Geometry check sheet. Reference: the model listing, model coordinates, mm. Face numbers are marked on the shaded views. A direction names the side the tool comes from. Coordinates: 2 decimals unless noted, no trailing zeros. Loops run counter-clockwise (first coordinate to the right, second up) from the corner with the lowest first, then second, coordinate; pieces in that order, holes last. Notation, with made-up numbers: (42.5, -15) -> (48.5, -15) arc R25 ccw to (48.5, -3) -> close; hole circle Ø1 at (-23.75, -13.75). An arc over 180 degrees is marked (long way). Answer as a JSON object with one key per item and string values.
from build123d import *

# Parameters (mm, degrees)
F0_W     = 440
F0_H     = 440
F1_DEPTH = 50.8
F0_W_2   = 50.8
F0_H_2   = 203.2
F0_W_3   = 203.2
F0_H_3   = 50.8
F2_DEPTH = 349.2
F3_DEPTH = 149.2
F4_W     = 440
F4_H     = 440
F4_W_2   = 50.8
F4_H_2   = 50.8
F5_DEPTH = 200


# Not quite as in the source:
# - a feature names something its author has since deleted; it is built from what else it names


with BuildPart() as f1:
    # F0 (on Top) → F1 (new body)
    with BuildSketch(Plane.XY):
        Polygon((91.7435496044, 289.8852448295), (-163.4564503956, 289.8852448295), (-163.4564503956, 239.0852448295), (-163.4564503956, 35.8852448295), (-214.2564503956, 35.8852448295), (-214.2564503956, -219.3147551705), (-163.4564503956, -219.3147551705), (39.7435496044, -219.3147551705), (39.7435496044, -270.1147551705), (294.9435496044, -270.1147551705), (294.9435496044, -219.3147551705), (294.9435496044, -16.1147551705), (345.7435496044, -16.1147551705), (345.7435496044, 239.0852448295), (294.9435496044, 239.0852448295), (91.7435496044, 239.0852448295), align=None)
        with Locations((65.7435496044, 9.8852448295)):
            Rectangle(F0_W, F0_H, mode=Mode.SUBTRACT)
        with Locations((65.7435496044, 9.8852448295)):
            Rectangle(F0_W, F0_H)
        Polygon((-65.0564503956, 140.6852448295), (-14.2564503956, 140.6852448295), (87.3435496044, 140.6852448295), (196.5435496044, 140.6852448295), (196.5435496044, 89.8852448295), (196.5435496044, -11.7147551705), (196.5435496044, -120.9147551705), (145.7435496044, -120.9147551705), (44.1435496044, -120.9147551705), (-65.0564503956, -120.9147551705), (-65.0564503956, -70.1147551705), (-65.0564503956, 31.4852448295), align=None, mode=Mode.SUBTRACT)
        Polygon((87.3435496044, 89.8852448295), (-14.2564503956, 89.8852448295), (-14.2564503956, 140.6852448295), (-65.0564503956, 140.6852448295), (-65.0564503956, 31.4852448295), (-14.2564503956, 31.4852448295), (-14.2564503956, -70.1147551705), (-65.0564503956, -70.1147551705), (-65.0564503956, -120.9147551705), (44.1435496044, -120.9147551705), (44.1435496044, -70.1147551705), (145.7435496044, -70.1147551705), (145.7435496044, -120.9147551705), (196.5435496044, -120.9147551705), (196.5435496044, -11.7147551705), (145.7435496044, -11.7147551705), (145.7435496044, 89.8852448295), (196.5435496044, 89.8852448295), (196.5435496044, 140.6852448295), (87.3435496044, 140.6852448295), align=None)
    extrude(amount=-F1_DEPTH)

    # F0 (on Top) → F2 (join)
    with BuildSketch(Plane.XY):
        Polygon((91.7435496044, 289.8852448295), (-163.4564503956, 289.8852448295), (-163.4564503956, 239.0852448295), (-163.4564503956, 35.8852448295), (-214.2564503956, 35.8852448295), (-214.2564503956, -219.3147551705), (-163.4564503956, -219.3147551705), (39.7435496044, -219.3147551705), (39.7435496044, -270.1147551705), (294.9435496044, -270.1147551705), (294.9435496044, -219.3147551705), (294.9435496044, -16.1147551705), (345.7435496044, -16.1147551705), (345.7435496044, 239.0852448295), (294.9435496044, 239.0852448295), (91.7435496044, 239.0852448295), align=None)
        with Locations((65.7435496044, 9.8852448295)):
            Rectangle(F0_W, F0_H, mode=Mode.SUBTRACT)
        with Locations((320.3435496044, -117.7147551705)):
            Rectangle(F0_W_2, F0_H_2)
        with Locations((193.3435496044, 264.4852448295)):
            Rectangle(F0_W_3, F0_H_3)
        with Locations((-188.8564503956, 137.4852448295)):
            Rectangle(F0_W_2, F0_H_2)
        with Locations((-61.8564503956, -244.7147551705)):
            Rectangle(F0_W_3, F0_H_3)
    extrude(amount=F2_DEPTH)

    # F0 (on Top) → F3 (join)
    with BuildSketch(Plane.XY):
        with Locations((65.7435496044, 9.8852448295)):
            Rectangle(F0_W, F0_H)
        Polygon((-65.0564503956, 140.6852448295), (-14.2564503956, 140.6852448295), (87.3435496044, 140.6852448295), (196.5435496044, 140.6852448295), (196.5435496044, 89.8852448295), (196.5435496044, -11.7147551705), (196.5435496044, -120.9147551705), (145.7435496044, -120.9147551705), (44.1435496044, -120.9147551705), (-65.0564503956, -120.9147551705), (-65.0564503956, -70.1147551705), (-65.0564503956, 31.4852448295), align=None, mode=Mode.SUBTRACT)
        Polygon((87.3435496044, 89.8852448295), (-14.2564503956, 89.8852448295), (-14.2564503956, 140.6852448295), (-65.0564503956, 140.6852448295), (-65.0564503956, 31.4852448295), (-14.2564503956, 31.4852448295), (-14.2564503956, -70.1147551705), (-65.0564503956, -70.1147551705), (-65.0564503956, -120.9147551705), (44.1435496044, -120.9147551705), (44.1435496044, -70.1147551705), (145.7435496044, -70.1147551705), (145.7435496044, -120.9147551705), (196.5435496044, -120.9147551705), (196.5435496044, -11.7147551705), (145.7435496044, -11.7147551705), (145.7435496044, 89.8852448295), (196.5435496044, 89.8852448295), (196.5435496044, 140.6852448295), (87.3435496044, 140.6852448295), align=None)
    extrude(amount=F3_DEPTH)

    # F4 (on face) → F5 (join)
    with BuildSketch(Plane.XY.offset(349.2)):
        Polygon((-163.4564503956, -219.3147551705), (-163.4564503956, -270.1147551705), (294.9435496044, -270.1147551705), (294.9435496044, -219.3147551705), (345.7435496044, -219.3147551705), (345.7435496044, 239.0852448295), (294.9435496044, 239.0852448295), (294.9435496044, 289.8852448295), (-163.4564503956, 289.8852448295), (-163.4564503956, 239.0852448295), (-214.2564503956, 239.0852448295), (-214.2564503956, -219.3147551705), align=None)
        with Locations((65.7435496044, 9.8852448295)):
            Rectangle(F4_W, F4_H, mode=Mode.SUBTRACT)
        with Locations((-188.8564503956, -244.7147551705)):
            Rectangle(F4_W_2, F4_H_2)
        with Locations((320.3435496044, 264.4852448295)):
            Rectangle(F4_W_2, F4_H_2)
        with Locations((-188.8564503956, 264.4852448295)):
            Rectangle(F4_W_2, F4_H_2)
        with Locations((320.3435496044, -244.7147551705)):
            Rectangle(F4_W_2, F4_H_2)
    extrude(amount=F5_DEPTH)


solid = f1.part
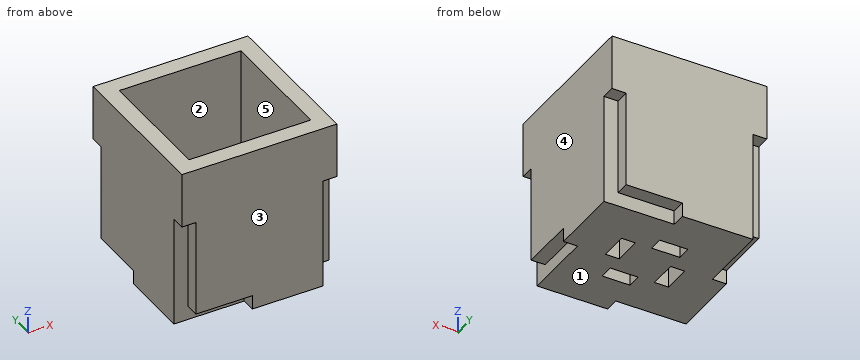
1. Section check B-B, the plane x = 8. Record the boundary of the cut face in (y, z), then the cut area to 3 significant figures.
Evaluation:
{"outline": "(-270.11, 0) -> (-219.31, 0) -> (-219.31, -50.8) -> (89.89, -50.8) -> (89.89, 149.2) -> (-210.11, 149.2) -> (-210.11, 549.2) -> (-270.11, 549.2) -> close; (140.69, -50.8) -> (289.89, -50.8) -> (289.89, 549.2) -> (229.89, 549.2) -> (229.89, 149.2) -> (140.69, 149.2) -> close", "area": "147,000 mm^2"}
2. Section check D-D, the plane y = -136.5. Record the boundary of the cut face in (x, z), then the cut area to 3 significant figures.
Evaluation:
{"outline": "(-214.26, -50.8) -> (294.94, -50.8) -> (294.94, 0) -> (345.74, 0) -> (345.74, 549.2) -> (285.74, 549.2) -> (285.74, 149.2) -> (-154.26, 149.2) -> (-154.26, 549.2) -> (-214.26, 549.2) -> close", "area": "157,000 mm^2"}
3. Depth check by flat-ended pin: P1, Ø6, axis at x = -84.5, y = 155, coming from the +Z side. Enter the tip coordinate at first touch or a pass-through.
Evaluation:
{"P1": "stops at z = 149.2"}
4. Mould release check, pull along Y, two halves, no side actions. Record for the marked faces 1, 2 and 3: released by +Y, released by -Y, zero draft, split by the parting line, or undercut.
Evaluation:
{"face 1": "zero draft", "face 2": "undercut", "face 3": "released by -Y"}
5. Section check C-C, the plane z = 60. Record the boundary of the cut face in (x, y).
Evaluation:
{"outline": "(-214.26, -219.31) -> (-163.46, -219.31) -> (-163.46, -270.11) -> (294.94, -270.11) -> (294.94, -219.31) -> (345.74, -219.31) -> (345.74, 239.09) -> (294.94, 239.09) -> (294.94, 289.89) -> (-163.46, 289.89) -> (-163.46, 239.09) -> (-214.26, 239.09) -> close; hole (-65.06, -70.11) -> (-14.26, -70.11) -> (-14.26, 31.49) -> (-65.06, 31.49) -> close; hole (-14.26, 89.89) -> (87.34, 89.89) -> (87.34, 140.69) -> (-14.26, 140.69) -> close; hole (44.14, -120.91) -> (145.74, -120.91) -> (145.74, -70.11) -> (44.14, -70.11) -> close; hole (145.74, -11.71) -> (196.54, -11.71) -> (196.54, 89.89) -> (145.74, 89.89) -> close"}
6. Section check A-A, the plane y = -27. Record the boundary of the cut face in (x, z).
Evaluation:
{"outline": "(-214.26, -50.8) -> (-65.06, -50.8) -> (-65.06, 149.2) -> (-154.26, 149.2) -> (-154.26, 549.2) -> (-214.26, 549.2) -> close; (-14.26, -50.8) -> (294.94, -50.8) -> (294.94, 0) -> (345.74, 0) -> (345.74, 549.2) -> (285.74, 549.2) -> (285.74, 149.2) -> (-14.26, 149.2) -> close"}
7. Thickness scan on probe 1 along Y at (x, z) = (55, -22.5); probe 2 along X at (y, z) = (26, -25.5); probe 3 along X at (y, z) = (-20, 447.5). Record the ranges inside material, lowest first. Write a range as from..to.
Evaluation:
{"probe 1": "y = -270.11..-120.91, -70.11..89.89, 140.69..289.89", "probe 2": "x = -214.26..-65.06, -14.26..145.74, 196.54..345.74", "probe 3": "x = -214.26..-154.26, 285.74..345.74"}
8. Tool access check on the marked faces 4 and 5. Record the directions out of +Z, -Z, +X, -X, +Y, -Y that give a thin tool (end or side, any length) a straight path to the whole face; none if there is none.
Evaluation:
{"face 4": "+Z, -Z, +X, +Y, -Y", "face 5": "+Z"}
